```python
from build123d import *

# Parameters (mm, degrees)
F1_DEPTH = 1.5


with BuildPart() as f1:
    # F0 (on Top) → F1 (new body)
    with BuildSketch(Plane.XY):
        with BuildLine():
            ThreePointArc((-19, 18), (-19.292893, 17.292893), (-20, 17))
            Line((-20, 17), (-20, -2))
            ThreePointArc((-20, -2), (-19.292893, -2.292893), (-19, -3))
            Line((-19, -3), (-19, -20.520575))
            ThreePointArc((-19, -20.520575), (-18.707107, -21.227682), (-18, -21.520575))
            ThreePointArc((-18, -21.520575), (-11.518915, -20.405966), (-5.782559, -17.190218))
            ThreePointArc((-5.782559, -17.190218), (-4.895494, -16.692937), (-3.893264, -16.520575))
            Line((-3.893264, -16.520575), (3.893264, -16.520575))
            ThreePointArc((3.893264, -16.520575), (4.895494, -16.692937), (5.782559, -17.190218))
            ThreePointArc((5.782559, -17.190218), (11.518915, -20.405966), (18, -21.520575))
            ThreePointArc((18, -21.520575), (18.707107, -21.227682), (19, -20.520575))
            Line((19, -20.520575), (19, -3))
            ThreePointArc((19, -3), (19.292893, -2.292893), (20, -2))
            Line((20, -2), (20, 17))
            ThreePointArc((20, 17), (19.292893, 17.292893), (19, 18))
            Line((19, 18), (19, 20.520575))
            ThreePointArc((19, 20.520575), (18.707107, 21.227682), (18, 21.520575))
            Line((18, 21.520575), (-18, 21.520575))
            ThreePointArc((-18, 21.520575), (-18.707107, 21.227682), (-19, 20.520575))
            Line((-19, 20.520575), (-19, 18))
        make_face()
        with BuildLine():
            Line((-11, -9.75), (11, -9.75))
            ThreePointArc((11, -9.75), (12.25, -11), (11, -12.25))
            Line((11, -12.25), (-11, -12.25))
            ThreePointArc((-11, -12.25), (-12.25, -11), (-11, -9.75))
        make_face(mode=Mode.SUBTRACT)
        with BuildLine():
            Line((-16.25, -8), (-16.25, 14))
            ThreePointArc((-16.25, 14), (-15, 15.25), (-13.75, 14))
            Line((-13.75, 14), (-13.75, -8))
            ThreePointArc((-13.75, -8), (-15, -9.25), (-16.25, -8))
        make_face(mode=Mode.SUBTRACT)
        with BuildLine():
            Line((4.25, -5.25), (-4.25, -5.25))
            ThreePointArc((-4.25, -5.25), (-7.785534, -3.785534), (-9.25, -0.25))
            Line((-9.25, -0.25), (-9.25, 6.25))
            ThreePointArc((-9.25, 6.25), (-7.785534, 9.785534), (-4.25, 11.25))
            Line((-4.25, 11.25), (4.25, 11.25))
            ThreePointArc((4.25, 11.25), (7.785534, 9.785534), (9.25, 6.25))
            Line((9.25, 6.25), (9.25, -0.25))
            ThreePointArc((9.25, -0.25), (7.785534, -3.785534), (4.25, -5.25))
        make_face(mode=Mode.SUBTRACT)
        with BuildLine():
            ThreePointArc((13.75, 14), (15, 15.25), (16.25, 14))
            Line((16.25, 14), (16.25, -8))
            ThreePointArc((16.25, -8), (15, -9.25), (13.75, -8))
            Line((13.75, -8), (13.75, 14))
        make_face(mode=Mode.SUBTRACT)
        with BuildLine():
            Line((-11, 18.25), (11, 18.25))
            ThreePointArc((11, 18.25), (12.25, 17), (11, 15.75))
            Line((11, 15.75), (-11, 15.75))
            ThreePointArc((-11, 15.75), (-12.25, 17), (-11, 18.25))
        make_face(mode=Mode.SUBTRACT)
    extrude(amount=F1_DEPTH)


solid = f1.part
```
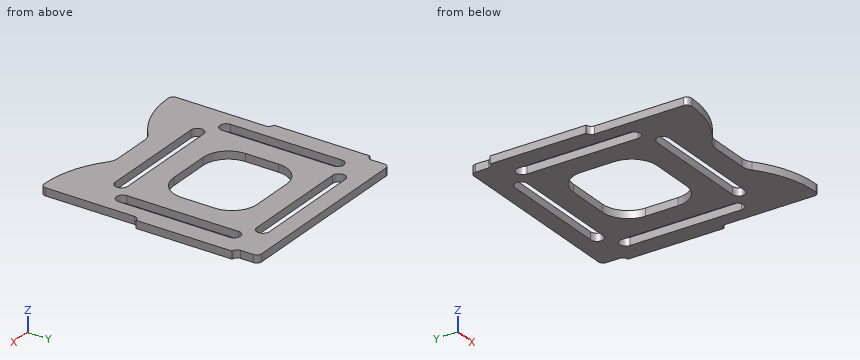
Check sheet for the modelled part. Datum: model origin and axes. Units: mm. Round coordinates to 2 decimals unless told otherwise and drop trailing zeros. Order: outer loops, then holes, each group sorted by start corner. A loop starts at its lowest first (then second) coordinate and runs counter-clockwise, first axis right, second up.
1) Section check C-C (y = 1.5). Record the boundary of the cut face in (x, z), and give its area (4 significant figures).
2) Section check B-B (x = 1). Record the boundary of the cut face in (y, z), and give its area (3 significant figures).
3) Section check A-A (y = -11). Record the boundary of the cut face in (x, z).
4) Go/stop test with a flat-tipped pin: pin 1 Ø0.8 at (x, z) = (3, 0.5) entering from -Y. Record where the tip stops, or that it passes through.
5) Scan lines: line 1 (X direction, y = -8, z = 0.75); line 2 (Y direction, x = -4, z = 0.6); line 3 (X direction, y = 2, z = 0.55). Record each from-to range of solid material in increasing order.
6) Section check D-D (x = 15). Record the boundary of the cut face in (y, z), and give its area (3 significant figures).
Result:
1. outline: (-20, 0) - (-16.25, 0) - (-16.25, 1.5) - (-20, 1.5) - close; (-13.75, 0) - (-9.25, 0) - (-9.25, 1.5) - (-13.75, 1.5) - close; (9.25, 0) - (13.75, 0) - (13.75, 1.5) - (9.25, 1.5) - close; (16.25, 0) - (20, 0) - (20, 1.5) - (16.25, 1.5) - close
1. area: 24.75 mm2
2. outline: (-16.52, 0) - (-12.25, 0) - (-12.25, 1.5) - (-16.52, 1.5) - close; (-9.75, 0) - (-5.25, 0) - (-5.25, 1.5) - (-9.75, 1.5) - close; (11.25, 0) - (15.75, 0) - (15.75, 1.5) - (11.25, 1.5) - close; (18.25, 0) - (21.52, 0) - (21.52, 1.5) - (18.25, 1.5) - close
2. area: 24.8 mm2
3. outline: (-19, 0) - (-12.25, 0) - (-12.25, 1.5) - (-19, 1.5) - close; (12.25, 0) - (19, 0) - (19, 1.5) - (12.25, 1.5) - close
4. pin 1: stops at y = -16.52
5. line 1: x = -19 to -16.25, -13.75 to 13.75, 16.25 to 19
5. line 2: y = -16.52 to -12.25, -9.75 to -5.25, 11.25 to 15.75, 18.25 to 21.52
5. line 3: x = -20 to -16.25, -13.75 to -9.25, 9.25 to 13.75, 16.25 to 20
6. outline: (-21.29, 0) - (-9.25, 0) - (-9.25, 1.5) - (-21.29, 1.5) - close; (15.25, 0) - (21.52, 0) - (21.52, 1.5) - (15.25, 1.5) - close
6. area: 27.5 mm2
